Here's how the part is built. I have some questions about the finished solid (model axes, mm). A direction names the side the tool comes from. Round coordinates to 2 decimals unless told otherwise and drop trailing zeros. Write each loop counter-clockwise with the first axis right and the second up, starting at its lowest first coordinate (ties: lowest second). Pieces come first, ordered by that corner, then holes. Notation, with made-up numbers: (46, -24.5) -> (103, -24.5) arc R34 ccw to (103, 5.5) -> close; hole circle Ø8 at (46, 39.5). An arc over 180 degrees is marked (long way). Put each result on its own line as item: value. Start each with the question number.
1. Suppose I cut it at A-A (y = -265). Please give me the cut outline in (x, z), then the cut area to 3 significant figures.
2. Which directions (+Z, -Z, +X, -X, +Y, -Y) give clear straight access to the entire face, cutting with the end or side of a thin tool? Please do faces 1 (the face through (-49.295, -221.987, 334.467)), 2 (the face through (266, 300.892, -63)), 3 (the face through (-269, -304.786, -63)), 4 (the face through (-305.159, -267, -63)), 5 (the face through (303.897, -267, -63)).
3. For pin 1 (3 mm diameter, centred on x = -69, y = 84, fed in from +Z); pin 2 (22.5 mm diameter, centred on x = 251.5, z = -89.5, fed in from +Y); pin 3 (22.5 mm diameter, centred on y = 273.5, z = -69, fed in from -X), each with a flat end and sliding along its axis, tell me the tip position at first contact or that it passes through.
4. Suppose I cut it at D-D (z = 439). Please give me the cut outline in (x, y).
5. Suppose I cut it at C-C (x = 0). Please give me the cut outline in (y, z), then the cut area to 3 significant figures.
6. Suppose I cut it at B-B (z = -73). Please give me the cut outline in (x, y).
7. We'd pull the mould along X, two halves only. Please class faces 6 (the face through (-230.856, 267, -63)), 7 (the face through (-4, 4, 0)), 8 (the face through (303.897, 264, -63)), 9 (the face through (-269, 303.144, -63)): +X half, -X half, draft (parallel to the pull), parting line (faces both ways), or undercut.
8. I need wall thicknesses on probe 1 along Y at (x, z) = (0, 335); probe 2 along Y at (x, z) = (290, 258); probe 3 along Z at (x, y) = (-6, -228.5). Which ranges of each line are inside material? Lowest first, please. Write a range as from..to.
```python
from build123d import *

# Parameters (mm, degrees)
F0_W      = 611.245334
F0_H      = 608.932316
F1_DEPTH  = 609.6
F3_W      = 729.550778
F3_H      = 731.767536
F4_DEPTH  = 25.4
F6_R      = 227.394025
F7_DEPTH  = 609.6
F9_W      = 74.302555
F9_H      = 74.302554
F9_W_2    = 74.302539
F9_H_2    = 74.302539
F10_DEPTH = 127


with BuildPart() as f1:
    # F0 (on Top) → F1 (new body)
    with BuildSketch(Plane.XY):
        Rectangle(F0_W, F0_H)
    extrude(amount=F1_DEPTH)

    # F3 (on offset) → F4 (join)
    with BuildSketch(Plane.XY.offset(609.6)):
        Rectangle(F3_W, F3_H)
    extrude(amount=F4_DEPTH)

    # F6 (on offset) → F7 (cut)
    with BuildSketch(Plane.XY.offset(635)):
        Circle(F6_R)
    extrude(amount=-F7_DEPTH, mode=Mode.SUBTRACT)

    # F9 (on offset) → F10 (join)
    with BuildSketch(Plane(origin=(0, 0, 0), x_dir=(1, 0, 0), z_dir=(0, 0, -1))):
        with Locations((-268.007428, 267.634988)):
            Rectangle(F9_W, F9_H)
        with Locations((266.745753, 267.634988)):
            Rectangle(F9_W_2, F9_H)
        with Locations((266.745753, -263.740815)):
            Rectangle(F9_W_2, F9_H_2)
        with Locations((-268.007428, -265.992411)):
            Rectangle(F9_W, F9_H_2)
    extrude(amount=F10_DEPTH)


solid = f1.part
```
Verdict:
1. outline: (-364.78, 609.6) -> (-305.62, 609.6) -> (-305.62, 0) -> (-305.16, 0) -> (-305.16, -127) -> (-230.86, -127) -> (-230.86, 0) -> (229.59, 0) -> (229.59, -127) -> (303.9, -127) -> (303.9, 0) -> (305.62, 0) -> (305.62, 609.6) -> (364.78, 609.6) -> (364.78, 635) -> (-364.78, 635) -> close
1. area: 410,000 mm^2
2. face 1: +Z
2. face 2: -Z, +X, +Y
2. face 3: -Z, +X, -X, -Y
2. face 4: -Z, -X, +Y, -Y
2. face 5: -Z, +X, +Y, -Y
3. pin 1: stops at z = 25.4
3. pin 2: stops at y = 300.89
3. pin 3: stops at x = -305.16
4. outline: (-305.62, -304.47) -> (305.62, -304.47) -> (305.62, 304.47) -> (-305.62, 304.47) -> close; hole circle Ø454.79 at (0, 0)
5. outline: (-365.88, 609.6) -> (-304.47, 609.6) -> (-304.47, 0) -> (304.47, 0) -> (304.47, 609.6) -> (365.88, 609.6) -> (365.88, 635) -> (227.39, 635) -> (227.39, 25.4) -> (-227.39, 25.4) -> (-227.39, 635) -> (-365.88, 635) -> close
5. area: 113,000 mm^2
6. outline: (-305.16, -304.79) -> (-230.86, -304.79) -> (-230.86, -230.48) -> (-305.16, -230.48) -> close; (-305.16, 228.84) -> (-230.86, 228.84) -> (-230.86, 303.14) -> (-305.16, 303.14) -> close; (229.59, -304.79) -> (303.9, -304.79) -> (303.9, -230.48) -> (229.59, -230.48) -> close; (229.59, 226.59) -> (303.9, 226.59) -> (303.9, 300.89) -> (229.59, 300.89) -> close
7. face 6: undercut
7. face 7: undercut
7. face 8: +X half
7. face 9: draft
8. probe 1: y = -304.47..-227.39, 227.39..304.47
8. probe 2: y = -304.47..304.47
8. probe 3: z = 0..635
